The model under review builds one solid part; all positions refer to its coordinate system, in mm. A direction names the side the tool comes from. Give positions to 0.01 mm unless a question says otherwise; leave off trailing zeros. Order: outer loops, then holes, each group sorted by start corner. A loop starts at its lowest first (then second) coordinate and runs counter-clockwise, first axis right, second up. Notation, with made-up numbers: (21, -22) - (65, -22) arc R15 ccw to (65, 5) - close; hole circle Ø8 at (47, -10.5). An arc over 180 degrees is marked (long way). Use CSV: the item, a comma, the result in double quotes.
Autodesk Inventor part; units mm, degrees
ref_plane "YZ Plane" through (0, 0, 0) normal (1, 0, 0) x (0, 1, 0)
ref_plane "XZ Plane" through (0, 0, 0) normal (0, 1, 0) x (-1, 0, 0)
ref_plane "XY Plane" through (0, 0, 0) normal (0, 0, 1) x (1, 0, 0)
sketch "Sketch2" plane through (0, 0, 0) normal (0, 1, 0) x (-1, 0, 0)
  arc A0 (3.5, 8.5) -> (1.5, 10.5) centre (1.5, 8.5) ccw
  arc A1 (1.5, -5.5) -> (3.5, -3.5) centre (1.5, -3.5) ccw
  line L0 (1.5, -5.5) -> (-1.5, -5.5)
  arc A2 (-3.5, -3.5) -> (-1.5, -5.5) centre (-1.5, -3.5) ccw
  arc A3 (-1.5, 10.5) -> (-3.5, 8.5) centre (-1.5, 8.5) ccw
  circle A4 centre (-9.4, -30.5) radius 1.7
  circle A5 centre (9.4, -15) radius 1.7
  circle A6 centre (9.4, 30.5) radius 1.7
  circle A7 centre (-9.4, 30.5) radius 1.7
  circle A8 centre (-9.4, 15) radius 1.7
  circle A9 centre (9.4, 15) radius 1.7
  circle A10 centre (-9.4, -15) radius 1.7
  circle A11 centre (9.4, -30.5) radius 1.7
  line L1 (-13.9, -33.875) -> (-13.9, 33.875)
  line L2 (13.9, -33.875) -> (-13.9, -33.875)
  line L3 (13.9, 33.875) -> (13.9, -33.875)
  line L4 (-13.9, 33.875) -> (13.9, 33.875)
  arc A12 (4.5, 8.5) -> (3.8682, 10.3417) centre (1.5, 8.5) ccw
  line L5 (-1.5, 10.5) -> (1.5, 10.5)
  arc A13 (-4.5, -3.5) -> (-1.5, -6.5) centre (-1.5, -3.5) ccw
  line L6 (-1.5, -6.5) -> (1.5, -6.5)
  arc A14 (1.5, -6.5) -> (4.5, -3.5) centre (1.5, -3.5) ccw
  arc A15 (4.5, 8.5) -> (1.5, 11.5) centre (1.5, 8.5) ccw
  line L7 (1.5, 11.5) -> (-1.5, 11.5)
  arc A16 (-1.5, 11.5) -> (-4.5, 8.5) centre (-1.5, 8.5) ccw
  line L8 (-1.5, 14.1) -> (1.5, 14.1)
  arc A17 (7.1, 8.5) -> (1.5, 14.1) centre (1.5, 8.5) ccw
  line L9 (7.1, 8.5) -> (7.1, -3.5)
  arc A18 (1.5, -9.1) -> (7.1, -3.5) centre (1.5, -3.5) ccw
  line L10 (1.5, -9.1) -> (-1.5, -9.1)
  arc A19 (-7.1, -3.5) -> (-1.5, -9.1) centre (-1.5, -3.5) ccw
  line L11 (-7.1, -3.5) -> (-7.1, 8.5)
  arc A20 (-1.5, 14.1) -> (-7.1, 8.5) centre (-1.5, 8.5) ccw
  line L12 (21.7007, 2.5) -> (-16.6227, 2.5) construction
  line L13 (4.9, 8.5) -> (4.9, 6.0503)
  arc A21 (1.5, -6.9) -> (4.9, -3.5) centre (1.5, -3.5) ccw
  line L14 (1.5, -6.9) -> (-1.5, -6.9)
  arc A22 (-4.9, -3.5) -> (-1.5, -6.9) centre (-1.5, -3.5) ccw
  line L15 (-4.9, 6.0503) -> (-4.9, 8.5)
  arc A23 (-1.5, 11.9) -> (-4.9, 8.5) centre (-1.5, 8.5) ccw
  line L16 (-1.5, 11.9) -> (1.5, 11.9)
  arc A24 (4.9, 8.5) -> (1.5, 11.9) centre (1.5, 8.5) ccw
  line L17 (6.7, -3.5) -> (6.7, 8.5)
  arc A25 (6.7, 8.5) -> (1.5, 13.7) centre (1.5, 8.5) ccw
  line L18 (1.5, 13.7) -> (-1.5, 13.7)
  arc A26 (-1.5, 13.7) -> (-6.7, 8.5) centre (-1.5, 8.5) ccw
  line L19 (-6.7, 8.5) -> (-6.7, -3.5)
  arc A27 (-6.7, -3.5) -> (-1.5, -8.7) centre (-1.5, -3.5) ccw
  line L20 (-1.5, -8.7) -> (1.5, -8.7)
  arc A28 (1.5, -8.7) -> (6.7, -3.5) centre (1.5, -3.5) ccw
  line L21 (2.9, 4.0503) -> (-2.9, 4.0503)
  line L22 (-2.9, 0.9497) -> (2.9, 0.9497)
  arc A29 (2.9, 4.0503) -> (4.9, 6.0503) centre (2.9, 6.0503) ccw
  arc A30 (-4.9, 6.0503) -> (-2.9, 4.0503) centre (-2.9, 6.0503) ccw
  line L23 (-4.9, -1.0503) -> (-4.9, -3.5)
  line L24 (4.9, -3.5) -> (4.9, -1.0503)
  arc A31 (4.9, -1.0503) -> (2.9, 0.9497) centre (2.9, -1.0503) ccw
  arc A32 (-2.9, 0.9497) -> (-4.9, -1.0503) centre (-2.9, -1.0503) ccw
  line L25 (-4.5, 8.5) -> (-4.5, 4.8503)
  line L26 (-4.5, 0.1497) -> (-4.5, -3.5)
  line L27 (-3.5, -3.5) -> (-3.5, 0.8576)
  line L28 (-3.5, 4.1424) -> (-3.5, 8.5)
  line L29 (3.5, 8.5) -> (3.5, 4.1424)
  line L30 (3.5, 0.8576) -> (3.5, -3.5)
  line L31 (4.5, -3.8243) -> (4.5, 0.1497)
  line L32 (4.5, 4.8503) -> (4.5, 8.5)
  line L33 (4.5, -3.5) -> (4.5, 0.1497)
  line L34 (4.5, 4.8503) -> (4.5, 8.5)
  circle A33 centre (-4.5, 2.5) radius 0.8
  circle A34 centre (4.5, 2.5) radius 0.8
  point P0 (0, 0)
  point P1 (0, 0)
  point P2 (2.621, 11.2827)
  point P3 (-2.6275, 11.2989)
  point P4 (3.8682, 10.3417)
  point P5 (4.5, 8.5)
  point P6 (4.5, -3.5)
  dimension "d10" = 2.6
  dimension "d11" = 23.2
  dimension "d12" = 14.2
  dimension "d15" = 23.2
  dimension "d17" = 0.4
  dimension "d18" = 2
  dimension "d19" = 2
  dimension "d20" = 1.6
  dimension "d21" = 1.6
  dimension "d22" = 2.2
  dimension "d23" = 2.2
extrude "Extrusion1" add sketch "Sketch2" along normal blind 1.5 contours A28 L20 A27 L19 A26 L18 A25 L17
equation "\"d23\" = d22"
properties part number "Top Seal 1"
Item 1: Tool access review of faces 4 (the face through (-6.7, 1, 2)), 5 (the face through (3.88, 0.74, -5.93)): name each direction out of +Z, -Z, +X, -X, +Y, -Y from which nothing blocks a thin tool from reaching the whole face with its end or side.
Results list:
face 4,"+Z, -Z, -X, +Y, -Y"
face 5,"+Y, -Y"
Item 2: Mouldability with a two-part tool opening along X and no side actions: class faces 1 (the face through (6.7, 1, 3)), 2 (the face through (0, 1, -8.7)), 3 (the face through (4.9, 1, -2)) as pulls with the +X half, pulls with the -X half, needs draft (parallel to the pull), parting line crosses it, or undercut.
Results list:
face 1,"pulls with the +X half"
face 2,"needs draft"
face 3,"undercut"
Item 3: Take a section at B-B, the plane x = 2.5. Give the boundary of the cut face in (y, z).
Results list:
outline,"(0, -8.6) - (1.5, -8.6) - (1.5, -6.75) - (0, -6.75) - close; (0, 0.95) - (1.5, 0.95) - (1.5, 4.05) - (0, 4.05) - close; (0, 11.75) - (1.5, 11.75) - (1.5, 13.6) - (0, 13.6) - close"
Item 4: Clearance check with flat-ended pins moving along their axes: pin 1 (8 mm diameter, centred on x = 4.5, z = -0.5, fed in from -Y); pin 2 (1 mm diameter, centred on x = -4.5, z = 2.5, fed in from +Y). State where each tip first meets the part, or that it passes through.
Results list:
pin 1,"stops at y = 0"
pin 2,"passes through"
Item 5: Wall thickness on L1, parallel to Z at x = -0.5, y = 0.55; L2, parallel to Z at x = 4.5, y = 0.9; L3, parallel to Z at x = 3, y = 0.6: over which ranges is each line inside the solid? List them lowest first.
Results list:
L1,"z = -8.7 to -6.9, 0.95 to 4.05, 11.9 to 13.7"
L2,"z = -7.75 to -5.1, 0.15 to 1.7, 3.3 to 4.85, 10.1 to 12.75"
L3,"z = -8.48 to -6.55, 0.95 to 4.05, 11.55 to 13.48"
Item 6: Take a section at C-C, the plane y = 1.1. Give the boundary of the cut face in (x, z), and give its area (3 significant figures).
Results list:
outline,"(-6.7, -3.5) arc R5.2 ccw to (-1.5, -8.7) - (1.5, -8.7) arc R5.2 ccw to (6.7, -3.5) - (6.7, 8.5) arc R5.2 ccw to (1.5, 13.7) - (-1.5, 13.7) arc R5.2 ccw to (-6.7, 8.5) - close; hole circle Ø1.6 at (-4.5, 2.5); hole (-4.9, -3.5) arc R3.4 ccw to (-1.5, -6.9) - (1.5, -6.9) arc R3.4 ccw to (4.9, -3.5) - (4.9, -1.05) arc R2 ccw to (2.9, 0.95) - (-2.9, 0.95) arc R2 ccw to (-4.9, -1.05) - close; hole (-4.9, 6.05) arc R2 ccw to (-2.9, 4.05) - (2.9, 4.05) arc R2 ccw to (4.9, 6.05) - (4.9, 8.5) arc R3.4 ccw to (1.5, 11.9) - (-1.5, 11.9) arc R3.4 ccw to (-4.9, 8.5) - close; hole circle Ø1.6 at (4.5, 2.5)"
area,"132 mm2"
Item 7: Take a section at D-D, the plane z = 2.5. Give the boundary of the cut face in (x, y), and give its area (3 significant figures).
Results list:
outline,"(-6.7, 0) - (-5.3, 0) - (-5.3, 1.5) - (-6.7, 1.5) - close; (-3.7, 0) - (3.7, 0) - (3.7, 1.5) - (-3.7, 1.5) - close; (5.3, 0) - (6.7, 0) - (6.7, 1.5) - (5.3, 1.5) - close"
area,"15.3 mm2"
Item 8: Take a section at A-A, the plane z = 7. Give the boundary of the cut face in (x, y).
Results list:
outline,"(-6.7, 0) - (-4.9, 0) - (-4.9, 1.5) - (-6.7, 1.5) - close; (4.9, 0) - (6.7, 0) - (6.7, 1.5) - (4.9, 1.5) - close"
